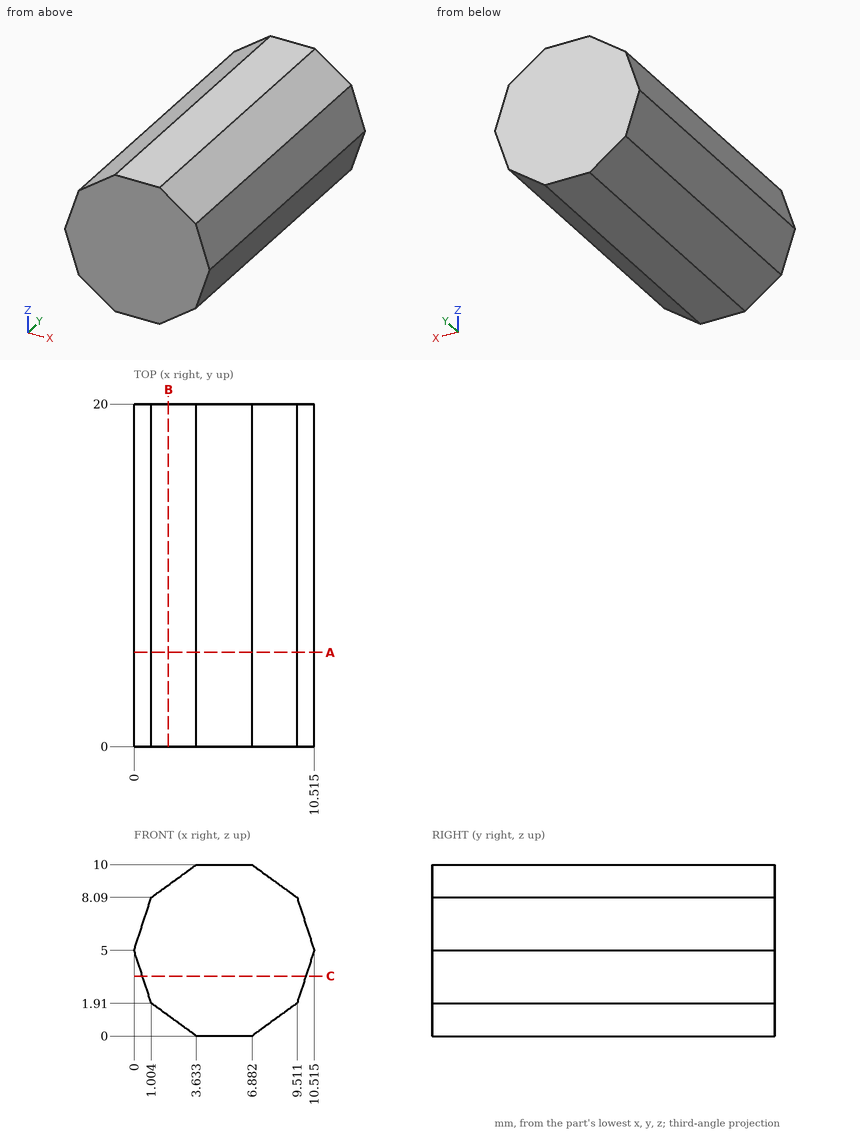
Can you work these out from the drawing? Everything is in mm from the part's minimum corner. Round coordinates to 2 decimals unless told otherwise and drop trailing zeros. Loops run counter-clockwise (first coordinate to the right, second up) from the corner with the lowest first, then second, coordinate; pieces in that order, holes last. Notation, with made-up numbers: (59.5, -18) - (108.5, -18) arc R17 ccw to (108.5, -8) - close; hole circle Ø3 at (43, 61). An arc over 180 degrees is marked (long way). Answer in a Markdown table with one row per item. Add a question column.
Q1. For pin 1 Ø6 at (y, z) = (5.5, 7.5) entering from -X; pin 2 Ø1 at (y, z) = (13, 4) entering from +X, each with a flat end and sliding along its axis, tell me the tip position at first contact or that it passes through.
Q2. I need wall thicknesses on L1, parallel to X at y = 14.5, z = 3.75 (1 decimal); L2, parallel to X at y = 7.25, z = 8.75 (1 decimal); L3, parallel to Z at x = 7.5, y = 13.75. Which ranges of each line are inside material? Lowest first, please.
Q3. I want a section at B-B on x = 2. List the corners of the cut face in (y, z) for me.
Q4. I want a section at C-C on z = 3.5. List the corners of the cut face in (x, y) for me, and give its area (3 significant figures).
Q5. I want a section at A-A on y = 5.5. List the corners of the cut face in (x, z) for me (1 decimal).
A:
| question | item | result |
|---|---|---|
| 1 | pin 1 | x = 0 |
| 1 | pin 2 | x = 10.35 |
| 2 | L1 | 0.4 to 10.1 |
| 2 | L2 | 1.9 to 8.6 |
| 2 | L3 | 0.45 to 9.55 |
| 3 | outline | (0, 1.19) - (20, 1.19) - (20, 8.81) - (0, 8.81) - close |
| 4 | outline | (0.49, 0) - (10.03, 0) - (10.03, 20) - (0.49, 20) - close |
| 4 | area | 191 mm^2 |
| 5 | outline | (0, 5) - (1, 1.9) - (3.6, 0) - (6.9, 0) - (9.5, 1.9) - (10.5, 5) - (9.5, 8.1) - (6.9, 10) - (3.6, 10) - (1, 8.1) - close |
